Read the model definition and answer for the solid it produces. Units are mm, in the model's axes. Coordinates: 2 decimals unless noted, no trailing zeros. Loops run counter-clockwise (first coordinate to the right, second up) from the corner with the lowest first, then second, coordinate; pieces in that order, holes last. Notation, with made-up numbers: (39, 51.25) -> (58, 51.25) arc R21 ccw to (58, 66.25) -> close; hole circle Ø10 at (11.25, 24). An arc over 180 degrees is marked (long way). Answer as CSV lines item,"result".
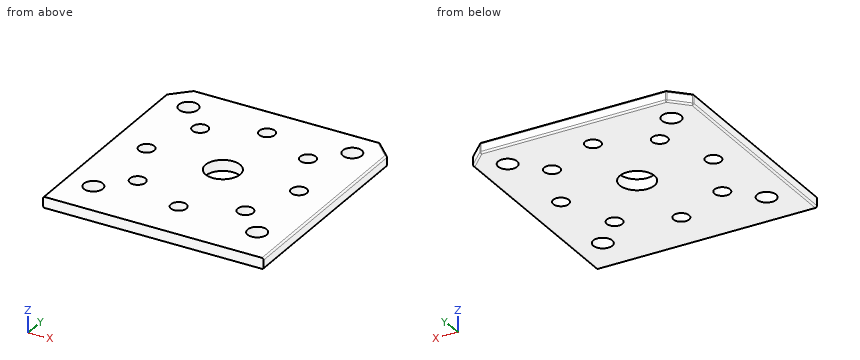
Autodesk Inventor part; units mm, degrees
ref_plane "YZ Plane" through (0, 0, 0) normal (1, 0, 0) x (0, 1, 0)
ref_plane "XZ Plane" through (0, 0, 0) normal (0, 1, 0) x (-1, 0, 0)
ref_plane "XY Plane" through (0, 0, 0) normal (0, 0, 1) x (1, 0, 0)
sketch "Sketch1" plane through (0, 0, 0) normal (0, 0, 1) x (1, 0, 0)
  line L0 (26.75, 31.75) -> (-26.75, 31.75)
  line L1 (-31.75, 26.75) -> (-31.75, -34.45)
  line L2 (-31.75, -34.45) -> (31.75, -34.45)
  line L3 (31.75, -34.45) -> (31.75, 26.75)
  circle A0 centre (0, 0) radius 5
  circle A1 centre (15.5, 15.5) radius 2.25
  circle A2 centre (-15.5, 15.5) radius 2.25
  circle A3 centre (-15.5, -15.5) radius 2.25
  circle A4 centre (15.5, -15.5) radius 2.25
  line L4 (-15.5, -15.5) -> (15.5, -15.5) construction
  line L5 (15.5, -15.5) -> (15.5, 15.5) construction
  line L6 (15.5, 15.5) -> (-15.5, 15.5) construction
  line L7 (-15.5, 15.5) -> (-15.5, -15.5) construction
  line L8 (0, 2.2207) -> (0, -2.8787) construction
  line L9 (-1.8221, 0) -> (3.1794, 0) construction
  circle A5 centre (0, 21.9203) radius 2.25
  circle A6 centre (0, -21.9203) radius 2.25
  circle A7 centre (-21.9203, 0) radius 2.25
  circle A8 centre (21.9203, 0) radius 2.25
  line L10 (0, 21.9203) -> (-21.9203, 0) construction
  line L11 (-21.9203, 0) -> (0, -21.9203) construction
  line L12 (0, -21.9203) -> (21.9203, 0) construction
  line L13 (21.9203, 0) -> (0, 21.9203) construction
  line L14 (-23.57, 23.57) -> (23.57, 23.57) construction
  line L15 (23.57, 23.57) -> (23.57, -23.57) construction
  line L16 (23.57, -23.57) -> (-23.57, -23.57) construction
  line L17 (-23.57, -23.57) -> (-23.57, 23.57) construction
  circle A9 centre (-23.57, 23.57) radius 2.75
  circle A10 centre (-23.57, -23.57) radius 2.75
  circle A11 centre (23.57, -23.57) radius 2.75
  circle A12 centre (23.57, 23.57) radius 2.75
  line L18 (-23.6, 28.2) -> (23.6, 28.2) construction
  line L19 (28.2, 23.6) -> (28.2, -23.6) construction
  line L20 (23.6, -28.2) -> (-23.6, -28.2) construction
  line L21 (-28.2, -23.6) -> (-28.2, 23.6) construction
  arc A13 (-23.6, 28.2) -> (-28.2, 23.6) centre (-23.6, 23.6) ccw construction
  arc A14 (-28.2, -23.6) -> (-23.6, -28.2) centre (-23.6, -23.6) ccw construction
  arc A15 (23.6, -28.2) -> (28.2, -23.6) centre (23.6, -23.6) ccw construction
  arc A16 (28.2, 23.6) -> (23.6, 28.2) centre (23.6, 23.6) ccw construction
  line L22 (-31.75, 26.75) -> (-26.75, 31.75)
  line L23 (26.75, 31.75) -> (31.75, 26.75)
  line L24 (-15.5, 21) -> (15.5, 21) construction
  line L25 (21, 15.5) -> (21, -15.5) construction
  line L26 (15.5, -21) -> (-15.5, -21) construction
  line L27 (-21, -15.5) -> (-21, 15.5) construction
  line L28 (-21, 15.5) -> (-15.5, 21) construction
  line L29 (15.5, 21) -> (21, 15.5) construction
  line L30 (21, -15.5) -> (15.5, -21) construction
  line L31 (-15.5, -21) -> (-21, -15.5) construction
  point P0 (-31.75, 31.75)
  point P1 (-31.75, 31.75)
  point P2 (31.75, 31.75)
  point P3 (28.2, -28.2)
  point P4 (-28.2, -28.2)
  point P5 (-31.75, 31.75)
  point P6 (31.75, 31.75)
  point P7 (-21, 21)
  point P8 (21, -21)
  point P9 (21, 21)
  point P10 (-21, -21)
  dimension "MotorPlateWidth" = 63.5
  dimension "MotorPlateHeight" = 66.2
  dimension "d5" = 31.75
  dimension "ShaftHole" = 10
  dimension "d10" = 4.5
  dimension "NEMA17HoleSpacing" = 31
  dimension "NEMA23HoleSpacing" = 47.14
  dimension "NEMA23MountingHole" = 5.5
  dimension "NEMA23Motor" = 56.4
  dimension "d35" = 4.6
  dimension "CornerChamfer" = 5
  dimension "d37" = 5
  dimension "d38" = 5
  dimension "d39" = 5
  dimension "NEMA17Motor" = 42
  dimension "NEMA17CornerChamfer" = 5.5
  dimension "d42" = 5.5
  dimension "d43" = 5.5
  dimension "d44" = 5.5
  dimension "d45" = 5.5
  dimension "d46" = 5.5
  dimension "d47" = 5.5
  dimension "d48" = 5.5
extrude "Extrusion1" add sketch "Sketch1" against normal blind 3.125
fillet "Fillet2" radius 0.5 14 edges at (-31.75, 26.75, -1.5625) (-29.25, 29.25, -3.125) (-26.75, 31.75, -1.5625) (0, 31.75, -3.125) (26.75, 31.75, -1.5625) (29.25, 29.25, -3.125) (31.75, 26.75, -1.5625) (-31.75, -3.85, -3.125) (31.75, -3.85, -3.125) (-29.25, 29.25, 0) (-31.75, -3.85, 0) (0, 31.75, 0) (29.25, 29.25, 0) (31.75, -3.85, 0)
equation "\"d10\" = NEMA17MountingHole"
properties part number "MOTOR001"
Q1. A cutting plane is placed at C-C, the plane x = 0. Write down the section's boundary in (y, z) (3 decimals), and give its area (3 significant figures).
Results:
outline,"(-34.45, -3.125) -> (-24.17, -3.125) -> (-24.17, 0) -> (-34.45, 0) -> close; (-19.67, -3.125) -> (-5, -3.125) -> (-5, 0) -> (-19.67, 0) -> close; (5, -3.125) -> (19.67, -3.125) -> (19.67, 0) -> (5, 0) -> close; (24.17, -3.125) -> (31.25, -3.125) arc R0.5 ccw to (31.75, -2.625) -> (31.75, -0.5) arc R0.5 ccw to (31.25, 0) -> (24.17, 0) -> close"
area,"147 mm²"
Q2. A cutting plane is placed at B-B, the plane y = 0. Write down the section's boundary in (x, z) (3 decimals), and give its area (3 significant figures).
Results:
outline,"(-31.75, -2.625) arc R0.5 ccw to (-31.25, -3.125) -> (-24.17, -3.125) -> (-24.17, 0) -> (-31.25, 0) arc R0.5 ccw to (-31.75, -0.5) -> close; (-19.67, -3.125) -> (-5, -3.125) -> (-5, 0) -> (-19.67, 0) -> close; (5, -3.125) -> (19.67, -3.125) -> (19.67, 0) -> (5, 0) -> close; (24.17, -3.125) -> (31.25, -3.125) arc R0.5 ccw to (31.75, -2.625) -> (31.75, -0.5) arc R0.5 ccw to (31.25, 0) -> (24.17, 0) -> close"
area,"139 mm²"
Q3. A cutting plane is placed at A-A, the plane y = 15.5. Write down the section's boundary in (x, z) (3 decimals), and give its area (3 significant figures).
Results:
outline,"(-31.75, -2.625) arc R0.5 ccw to (-31.25, -3.125) -> (-17.75, -3.125) -> (-17.75, 0) -> (-31.25, 0) arc R0.5 ccw to (-31.75, -0.5) -> close; (-13.25, -3.125) -> (13.25, -3.125) -> (13.25, 0) -> (-13.25, 0) -> close; (17.75, -3.125) -> (31.25, -3.125) arc R0.5 ccw to (31.75, -2.625) -> (31.75, -0.5) arc R0.5 ccw to (31.25, 0) -> (17.75, 0) -> close"
area,"170 mm²"
Q4. A cutting plane is placed at D-D, the plane z = -1.3. Give the number of separate pieces and of enclosed holes in the cut face, and give its area (3 significant figures).
Results:
separate pieces,"1"
enclosed holes,"13"
area,"3,880 mm²"
Q5. Find the intervals of material crossed by probe 1 along Y at (x, z) = (0, -1.65); probe 2 along Y at (x, z) = (-1, -1.25); probe 3 along Y at (x, z) = (15.5, -1.5), in increasing order. Write a range as [from, to].
Results:
probe 1,"y = [-34.45, -24.17], [-19.67, -5], [5, 19.67], [24.17, 31.75]"
probe 2,"y = [-34.45, -23.94], [-19.9, -4.9], [4.9, 19.9], [23.94, 31.75]"
probe 3,"y = [-34.45, -17.75], [-13.25, 13.25], [17.75, 31.75]"
